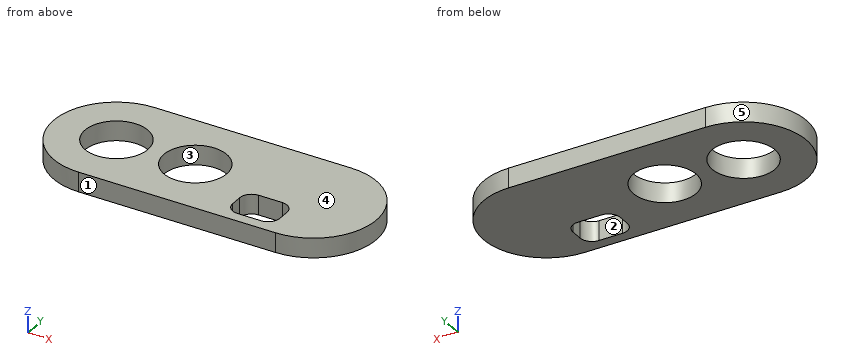
from build123d import *

# Parameters (mm, degrees)
SKETCH_1_R      = 8
EXTRUDE_1_DEPTH = 5


with BuildPart() as part:
    # 草图1 → 凸台-拉伸1 (new body)
    with BuildSketch(Plane.XY):
        with BuildLine():
            ThreePointArc((-21.649032952, 39.411076993), (-37.649032952, 23.411076993), (-21.649032952, 7.411076993))
            Line((-21.649032952, 7.411076993), (28.350967048, 7.411076993))
            ThreePointArc((28.350967048, 7.411076993), (44.350967048, 23.411076993), (28.350967048, 39.411076993))
            Line((28.350967048, 39.411076993), (-21.649032952, 39.411076993))
        make_face()
        with Locations((-21.649032952, 23.411076993)):
            Circle(SKETCH_1_R, mode=Mode.SUBTRACT)
        with Locations((-1.649032952, 23.411076993)):
            Circle(SKETCH_1_R, mode=Mode.SUBTRACT)
        with BuildLine():
            ThreePointArc((16.970957649, 10.16166095), (14.849637306, 11.040340606), (13.970957649, 13.16166095))
            Line((13.970957649, 13.16166095), (13.970957649, 16.16166095))
            ThreePointArc((13.970957649, 16.16166095), (14.849637306, 18.282981293), (16.970957649, 19.16166095))
            Line((16.970957649, 19.16166095), (22.970957649, 19.16166095))
            ThreePointArc((22.970957649, 19.16166095), (25.092277993, 18.282981293), (25.970957649, 16.16166095))
            Line((25.970957649, 16.16166095), (25.970957649, 13.16166095))
            ThreePointArc((25.970957649, 13.16166095), (25.092277993, 11.040340606), (22.970957649, 10.16166095))
            Line((22.970957649, 10.16166095), (16.970957649, 10.16166095))
        make_face(mode=Mode.SUBTRACT)
    extrude(amount=EXTRUDE_1_DEPTH)


solid = part.part
Source: CAD feature listing. Evaluate the final solid. Frame: model axes, mm. Face numbers are marked on the shaded views. A direction names the side the tool comes from. Give positions to 0.01 mm unless a question says otherwise; leave off trailing zeros. Write each loop counter-clockwise with the first axis right and the second up, starting at its lowest first coordinate (ties: lowest second). Pieces come first, ordered by that corner, then holes. Notation, with made-up numbers: (-8.75, 23.5) - (28.25, 23.5) arc R24 ccw to (28.25, 35.5) - close; hole circle Ø5 at (53, 42.5). An arc over 180 degrees is marked (long way). Write item = value, one per line. Start each with the question number.
Q1. Reachability of the marked faces 1 and 2 from +Z, -Z, +X, -X, +Y, -Y: full face, straight path, thin tool, end or side. Return the list, or none.
Q2. Cut plane B-B, the plane z = 1.95. Return loops of the section in (x, y), then the cut area to 3 significant figures.
Q3. Cut plane A-A, the plane y = 12. Return loops of the section in (x, z) (3 decimals), then the cut area to 3 significant figures.
Q4. Pin query (flat end, axial travel): pin 1 Ø1.5 at (x, y) = (11, 18) entering from -Z; pin 2 Ø2.5 at (y, z) = (15.5, 1.5) entering from -X; pin 3 Ø0.9 at (y, z) = (14, 3) entering from +X. Return the tip coordinate at first contact, or that it passes through.
Q5. Draft query along Y for the marked faces 3, 4 and 5. Return one class per face: +Y half, -Y half, draft (parallel to the pull), parting line (faces both ways), or undercut.
Q6. Cut plane C-C, the plane y = 17. Return loops of the section in (x, z), then the cut area to 3 significant figures.
Q7. Cut plane D-D, the plane x = -7.5. Return loops of the section in (y, z), then the cut area to 3 significant figures.
Q8. Material intervals for probe 1 along X at (y, z) = (23, 0.4); probe 2 along X at (y, z) = (29.5, 0.5); probe 3 along Y at (x, z) = (-3.5, 3.9), sorted ascending.
Computed values:
q1.face_1 = +Z, -Z, +X, -X, -Y
q1.face_2 = +Z, -Z
q2.outline = (-21.65, 7.41) - (28.35, 7.41) arc R16 ccw to (28.35, 39.41) - (-21.65, 39.41) arc R16 ccw to start; hole circle Ø16 at (-21.65, 23.41); hole circle Ø16 at (-1.65, 23.41); hole (13.97, 13.16) arc R3 ccw to (16.97, 10.16) - (22.97, 10.16) arc R3 ccw to (25.97, 13.16) - (25.97, 16.16) arc R3 ccw to (22.97, 19.16) - (16.97, 19.16) arc R3 ccw to (13.97, 16.16) - close
q2.area = 1,900 mm²
q3.outline = (-32.865, 0) - (14.205, 0) - (14.205, 5) - (-32.865, 5) - close; (25.737, 0) - (39.566, 0) - (39.566, 5) - (25.737, 5) - close
q3.area = 304 mm²
q4.pin_1 = 0
q4.pin_2 = -36.2
q4.pin_3 = 41.61
q5.face_3 = undercut
q5.face_4 = draft
q5.face_5 = parting line
q6.outline = (-36.31, 0) - (-26.43, 0) - (-26.43, 5) - (-36.31, 5) - close; (-16.86, 0) - (-6.43, 0) - (-6.43, 5) - (-16.86, 5) - close; (3.14, 0) - (14.09, 0) - (14.09, 5) - (3.14, 5) - close; (25.85, 0) - (43.01, 0) - (43.01, 5) - (25.85, 5) - close
q6.area = 242 mm²
q7.outline = (7.41, 0) - (17.96, 0) - (17.96, 5) - (7.41, 5) - close; (28.87, 0) - (39.41, 0) - (39.41, 5) - (28.87, 5) - close
q7.area = 105 mm²
q8.probe_1 = -37.64 to -29.64, -13.66 to -9.64, 6.34 to 44.35
q8.probe_2 = -36.45 to -26.84, -16.46 to -6.84, 3.54 to 43.15
q8.probe_3 = 7.41 to 15.63, 31.19 to 39.41
